Could you check a few things on this model? Use its own coordinates, in mm. Face numbers are marked on the shaded views. A direction names the side the tool comes from. Coordinates: 2 decimals unless noted, no trailing zeros. Loops run counter-clockwise (first coordinate to the right, second up) from the corner with the lowest first, then second, coordinate; pieces in that order, holes last.
1) Imagine slicing it at A-A on z = 0. Please give me the cut outline in (x, y).
2) Will these pins go through, and if not, where does the flat tip stop? P1, Ø2, axis at y = 1, z = 0, coming from the +X side; P2, Ø3, axis at x = -46, z = 1, coming from the +Y side; P3, Ø0.5, axis at y = 3, z = -0.5, coming from the -X side.
3) For the marked faces 1, 2 and 3, which set-ups out of +Z, -Z, +X, -X, +Y, -Y let a thin tool reach every point of the face, with its end or its side?
4) Imagine slicing it at D-D on x = -3.5. Please give me the cut outline in (y, z), plus the area to 3 significant figures.
5) Imagine slicing it at B-B on y = 0. Please give me the cut outline in (x, z), plus the area to 3 significant figures.
6) Imagine slicing it at C-C on x = -49. Please give me the cut outline in (y, z).
7) Thinking about a two-plate mould opening in X: for the marked faces 4, 5, 6 and 7, which applies, released by +X, released by -X, zero draft, split by the parting line, or undercut?
8) If I drill on line 1 along X through (y, z) = (-1, 0); line 2 along Y through (x, z) = (-3.5, 1.5); line 3 along X through (y, z) = (-1.75, -3), over which ranges is the centre line in solid material (lowest first)?
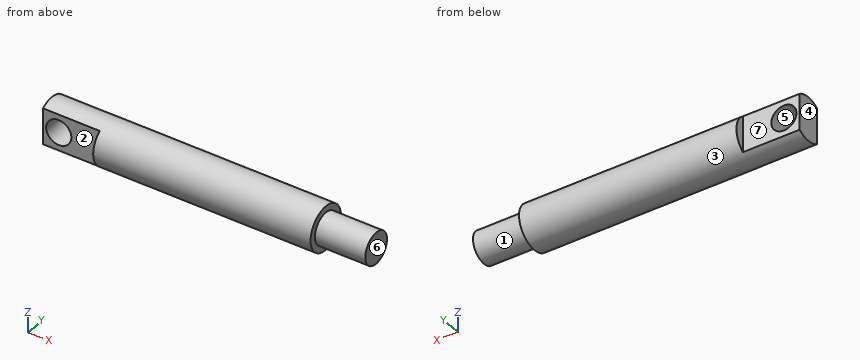
Autodesk Inventor part; units mm, degrees
ref_plane "YZ Plane" through (0, 0, 0) normal (1, 0, 0) x (0, 1, 0)
ref_plane "XZ Plane" through (0, 0, 0) normal (0, 1, 0) x (-1, 0, 0)
ref_plane "XY Plane" through (0, 0, 0) normal (0, 0, 1) x (1, 0, 0)
sketch "Sketch1" plane through (0, 0, 0) normal (0, 0, 1) x (1, 0, 0)
  line L0 (0, 0) -> (0, 2.5)
  line L1 (0, 2.5) -> (-8, 2.5)
  line L2 (-8, 2.5) -> (-8, 3.5)
  line L3 (-8, 3.5) -> (-51.5, 3.5)
  line L4 (-51.5, 3.5) -> (-51.5, 0)
  line L5 (-51.5, 0) -> (0, 0)
  point P0 (-4, 2.5)
  dimension "d0" = 5
  dimension "d1" = 7
  dimension "d2" = 8
  dimension "d19" = 43.5
revolve "Revolution1" add sketch "Sketch1" angle 360 about axis through (-51.5, 0, 0) along (1, 0, 0)
thread "Thread1"
sketch "Sketch3" plane through (-51.5, 0, 0) normal (-1, 0, 0) x (0, 0, 1)
  circle A0 centre (0, 0) radius 3.5
  line L0 (-2.8723, 2) -> (2.8723, 2)
  circle A1 centre (0, 0) radius 3.5
  line L1 (-2.8723, -2) -> (2.8723, -2)
  arc A2 (-2.8723, 2) -> (-2.8723, -2) centre (0, 0) ccw
  arc A3 (2.8723, -2) -> (2.8723, 2) centre (0, 0) ccw
  point P0 (0, 0)
  dimension "d7" = 2
  dimension "d8" = 2
extrude "Extrusion1" cut sketch "Sketch3" against normal blind 9 contours L0 A0 | A0 L1
sketch "Sketch4" plane through (-51.5, -2, -2.8723) normal (0, -1, 0) x (1, 0, 0)
  line L0 (0, 0) -> (0, 5.7446)
  point P0 (51.5, 2.8723)
  point P1 (2.5, 2.8723)
  point P2 (0, 2.8723)
  dimension "d11" = 2.5
hole "Hole1" at (-49, -2, 0) direction (0, 1, 0) diameter 4 depth 4
properties part number "11 fitting"
Filled in:
1. outline: (-51.5, -2) - (-51, -2) - (-51, 2) - (-51.5, 2) - close; (-47, -2) - (-42.5, -2) - (-42.5, -3.5) - (-8, -3.5) - (-8, -2.5) - (0, -2.5) - (0, 2.5) - (-8, 2.5) - (-8, 3.5) - (-42.5, 3.5) - (-42.5, 2) - (-47, 2) - close
2. P1: stops at x = 0
2. P2: stops at y = 2
2. P3: stops at x = -42.5
3. face 1: +X
3. face 2: +Z, -Z, -X, -Y
3. face 3: +X, -X
4. outline: circle Ø5 at (0, 0)
4. area: 19.6 mm2
5. outline: (-51.5, -3.5) - (-8, -3.5) - (-8, -2.5) - (0, -2.5) - (0, 2.5) - (-8, 2.5) - (-8, 3.5) - (-51.5, 3.5) - close; hole circle Ø4 at (-49, 0)
5. area: 332 mm2
6. outline: (-2, -2.87) arc R3.5 ccw to (2, -2.87) - (2, -2) - (-2, -2) - close; (-2, 2) - (2, 2) - (2, 2.87) arc R3.5 ccw to (-2, 2.87) - close
7. face 4: released by -X
7. face 5: undercut
7. face 6: released by +X
7. face 7: zero draft
8. line 1: x = -51.5 to -51, -47 to 0
8. line 2: y = -2 to 2
8. line 3: x = -51.5 to -8
